```python
from build123d import *

# Parameters (mm, degrees)
F0_W     = 508
F0_H     = 457.2
F1_DEPTH = 12.7
F2_W     = 30.48
F2_H     = 63.5
F3_DEPTH = 5.08
F2_R     = 12.7
F4_DEPTH = 5.08
F2_W_2   = 55.88
F2_H_2   = 30.48
F5_DEPTH = 12.7


with BuildPart() as f1:
    # F0 (on Front) → F1 (new body)
    with BuildSketch(Plane.XZ):
        with Locations((16.225851, -9.961791)):
            Rectangle(F0_W, F0_H)
    extrude(amount=F1_DEPTH)

    # F2 (on face) → F3 (cut)
    with BuildSketch(Plane.XZ.offset(12.7)):
        with Locations((158.465851, -181.411791)):
            Rectangle(F2_W, F2_H)
        with Locations((-126.014149, -181.411791)):
            Rectangle(F2_W, F2_H)
    extrude(amount=-F3_DEPTH, mode=Mode.SUBTRACT)

    # F2 (on face) → F4 (cut)
    with BuildSketch(Plane.XZ.offset(12.7)):
        with Locations((-208.564149, 180.538209)):
            Circle(F2_R)
        with Locations((243.555851, 180.538209)):
            Circle(F2_R)
    extrude(amount=-F4_DEPTH, mode=Mode.SUBTRACT)

    # F2 (on face) → F5 (cut)
    with BuildSketch(Plane.XZ.offset(12.7)):
        with Locations((16.225851, -223.321791)):
            Rectangle(F2_W_2, F2_H_2)
    extrude(amount=-F5_DEPTH, mode=Mode.SUBTRACT)


solid = f1.part
```
Part model, mm, in its own coordinate system. A direction names the side the tool comes from. Round coordinates to 2 decimals unless told otherwise and drop trailing zeros. Write each loop counter-clockwise with the first axis right and the second up, starting at its lowest first coordinate (ties: lowest second). Pieces come first, ordered by that corner, then holes. Notation, with made-up numbers: (37.5, 49) -> (43.5, 49) arc R33 ccw to (43.5, 83) -> close; hole circle Ø7 at (88, 43.25). An arc over 180 degrees is marked (long way). Return JSON: item names as keys, results as strings. Group by question number.
Q1. Pin check, flat tips, straight feed: pin 1 (4 mm diameter, centred on x = 27.5, y = -8, fed in from -Z); pin 2 (15 mm diameter, centred on x = -208.56, z = 180.54, fed in from -Y). Stop position of each tip, or through.
Q2. Saw through at A-A on z = -198. Write the cut outline in (x, y), plus the area to 3 significant figures.
Q3. Which spindle directions (+Z, -Z, +X, -X, +Y, -Y) get a long thin tool onto all of the face, cutting with end or side? Do faces 1 (the flat face through (-126, -7.62, -181)), 2 (the flat face through (44.166, -6, -224)), 3 (the flat face through (-237.774, -6, -13)). Say none if no direction does.
Q4. Mould opens along X. For faces 4 (the flat face through (270.226, -6, -13)), 5 (the flat face through (13, -12.7, -7)), 6 (the cylindrical face through (-196.833, -10.196, 175.674)) say: pulls with the +X half, pulls with the -X half, needs draft (parallel to the pull), parting line crosses it, or undercut.
Q5. Probe L1, parallel to Z at x = -121.5, y = -9.75; L2, parallel to Z at x = -1.5, y = -6.5; L3, parallel to Y at x = -117.5, z = -211.5. List the from-to ranges inside material, lowest first. Write a range as [from, to].
Q6. Saw through at B-B on x = 4. Write the cut outline in (y, z), plus the area to 3 significant figures.
Answer:
{
 "1": {"pin 1": "z = -208.08", "pin 2": "y = -7.62"},
 "2": {"outline": "(-237.77, -12.7) -> (-141.25, -12.7) -> (-141.25, -7.62) -> (-110.77, -7.62) -> (-110.77, -12.7) -> (143.23, -12.7) -> (143.23, -7.62) -> (173.71, -7.62) -> (173.71, -12.7) -> (270.23, -12.7) -> (270.23, 0) -> (-237.77, 0) -> close", "area": "6,140 mm2"},
 "3": {"face 1": "-Y", "face 2": "-Z, +Y, -Y", "face 3": "+Z, -Z, -X, +Y, -Y"},
 "4": {"face 4": "pulls with the +X half", "face 5": "needs draft", "face 6": "undercut"},
 "5": {"L1": "[-238.56, -213.16], [-149.66, 218.64]", "L2": "[-208.08, 218.64]", "L3": "[-7.62, 0]"},
 "6": {"outline": "(-12.7, -208.08) -> (0, -208.08) -> (0, 218.64) -> (-12.7, 218.64) -> close", "area": "5,420 mm2"}
}
